from build123d import *

# Parameters (mm, degrees)
SKETCH_1_W                = 23.5
SKETCH_1_H                = 12
EXTRUDE_1_DEPTH           = 510.5
HOLE_WIZARD_M6_1_D        = 5
HOLE_WIZARD_M6_1_DEPTH    = 19
HOLE_WIZARD_M6_1_TIP      = 1.502151548
HOLE_WIZARD_M6_2_D        = 5
HOLE_WIZARD_M6_2_DEPTH    = 15
HOLE_WIZARD_M6_2_TIP      = 1.502151548
HOLE_WIZARD_9_0_9_1_D     = 9
HOLE_WIZARD_M6_3_D        = 5
HOLE_WIZARD_M6_3_DEPTH    = 15
HOLE_WIZARD_M6_3_TIP      = 1.502151548
HOLE_WIZARD_9_0_9_2_D     = 9
HOLE_WIZARD_7_0_7_1_D     = 7
HOLE_WIZARD_7_0_7_1_DEPTH = 15
HOLE_WIZARD_7_0_7_1_TIP   = 2.103012167
HOLE_WIZARD_M6_4_D        = 5
HOLE_WIZARD_M6_4_DEPTH    = 17
HOLE_WIZARD_M6_4_TIP      = 1.502151548


with BuildPart() as part:
    # 草图1 → 凸台-拉伸1 (new, symmetric)
    with BuildSketch(Plane(origin=(0, 0, 0), x_dir=(0, 0, -1), z_dir=(1, 0, 0))):
        Polygon((-15, 15), (-11.5, 15), (-11.5, 13.5), (-11, 13.5), (-11, 12), (-9.5, 12), (-9.5, 15), (-8, 15), (-8, 12.5), (-5, 12.5), (-5, 15), (5, 15), (5, 12.5), (8, 12.5), (8, 15), (9.5, 15), (9.5, 12), (11, 12), (11, 13.5), (11.5, 13.5), (11.5, 15), (15, 15), (15, 8), (12.5, 8), (12.5, 5), (15, 5), (15, -5), (12.5, -5), (12.5, -8), (15, -8), (15, -15), (11.5, -15), (11.5, -13.5), (11, -13.5), (11, -12), (9.5, -12), (9.5, -15), (8, -15), (8, -12.5), (5, -12.5), (5, -15), (-5, -15), (-5, -12.5), (-8, -12.5), (-8, -15), (-9.5, -15), (-9.5, -12), (-11, -12), (-11, -13.5), (-11.5, -13.5), (-11.5, -15), (-15, -15), align=None)
        with BuildLine():
            Line((12, -10.5), (12, -8.5))
            ThreePointArc((12, -8.5), (11.853553391, -8.146446609), (11.5, -8))
            Line((11.5, -8), (-11.5, -8))
            ThreePointArc((-11.5, -8), (-11.853553391, -8.146446609), (-12, -8.5))
            Line((-12, -8.5), (-12, -10.5))
            ThreePointArc((-12, -10.5), (-11.853553391, -10.853553391), (-11.5, -11))
            Line((-11.5, -11), (11.5, -11))
            ThreePointArc((11.5, -11), (11.853553391, -10.853553391), (12, -10.5))
        make_face(mode=Mode.SUBTRACT)
        with BuildLine():
            Line((-11.5, 11), (11.5, 11))
            ThreePointArc((11.5, 11), (11.853553391, 10.853553391), (12, 10.5))
            Line((12, 10.5), (12, 8.5))
            ThreePointArc((12, 8.5), (11.853553391, 8.146446609), (11.5, 8))
            Line((11.5, 8), (-11.5, 8))
            ThreePointArc((-11.5, 8), (-11.853553391, 8.146446609), (-12, 8.5))
            Line((-12, 8.5), (-12, 10.5))
            ThreePointArc((-12, 10.5), (-11.853553391, 10.853553391), (-11.5, 11))
        make_face(mode=Mode.SUBTRACT)
        Rectangle(SKETCH_1_W, SKETCH_1_H, mode=Mode.SUBTRACT)
    extrude(amount=EXTRUDE_1_DEPTH, both=True)

    # M6 螺纹孔1
    with Locations(Plane(origin=(0, 0, -15), x_dir=(-1, 0, 0), z_dir=(0, 0, -1))):
        with Locations((460.5, 0), (445.5, 0), (-445.5, 0), (-460.5, 0)):
            Hole(HOLE_WIZARD_M6_1_D / 2, depth=HOLE_WIZARD_M6_1_DEPTH)
            with Locations((0, 0, -(HOLE_WIZARD_M6_1_DEPTH + HOLE_WIZARD_M6_1_TIP / 2))):  # 118° drill point
                Cone(0, HOLE_WIZARD_M6_1_D / 2, HOLE_WIZARD_M6_1_TIP, mode=Mode.SUBTRACT)

    # M6 螺纹孔2
    with Locations(Plane(origin=(0, -15, 0), x_dir=(-1, 0, 0), z_dir=(0, -1, 0))):
        with Locations((-460.5, 0), (-445.5, 0), (215.5, 0), (230.5, 0), (445.5, 0), (460.5, 0)):
            Hole(HOLE_WIZARD_M6_2_D / 2, depth=HOLE_WIZARD_M6_2_DEPTH)
            with Locations((0, 0, -(HOLE_WIZARD_M6_2_DEPTH + HOLE_WIZARD_M6_2_TIP / 2))):  # 118° drill point
                Cone(0, HOLE_WIZARD_M6_2_D / 2, HOLE_WIZARD_M6_2_TIP, mode=Mode.SUBTRACT)

    # Ø9.0 (9) 直径孔1 (through all)
    with Locations(Plane.XY.offset(15)):
        with Locations((-422.5, 0), (422.5, 0)):
            Hole(HOLE_WIZARD_9_0_9_1_D / 2)

    # M6 螺纹孔3
    with Locations(Plane(origin=(0, 15, 0), x_dir=(1, 0, 0), z_dir=(0, 1, 0))):
        with Locations((-355.5, 0), (400.5, 0)):
            Hole(HOLE_WIZARD_M6_3_D / 2, depth=HOLE_WIZARD_M6_3_DEPTH)
            with Locations((0, 0, -(HOLE_WIZARD_M6_3_DEPTH + HOLE_WIZARD_M6_3_TIP / 2))):  # 118° drill point
                Cone(0, HOLE_WIZARD_M6_3_D / 2, HOLE_WIZARD_M6_3_TIP, mode=Mode.SUBTRACT)

    # Ø9.0 (9) 直径孔2 (through all)
    with Locations(Plane(origin=(0, -15, 0), x_dir=(-1, 0, 0), z_dir=(0, -1, 0))):
        with Locations((-183, 0), (390.5, 0)):
            Hole(HOLE_WIZARD_9_0_9_2_D / 2)

    # Ø7.0 (7) 直径孔1
    with Locations(Plane(origin=(0, -15, 0), x_dir=(-1, 0, 0), z_dir=(0, -1, 0))):
        with Locations((-400.5, 0), (355.5, 0)):
            Hole(HOLE_WIZARD_7_0_7_1_D / 2, depth=HOLE_WIZARD_7_0_7_1_DEPTH)
            with Locations((0, 0, -(HOLE_WIZARD_7_0_7_1_DEPTH + HOLE_WIZARD_7_0_7_1_TIP / 2))):  # 118° drill point
                Cone(0, HOLE_WIZARD_7_0_7_1_D / 2, HOLE_WIZARD_7_0_7_1_TIP, mode=Mode.SUBTRACT)

    # M6 螺纹孔4
    with Locations(Plane(origin=(0, 0, -15), x_dir=(-1, 0, 0), z_dir=(0, 0, -1))):
        with Locations((-368.5, 0), (-298.499999898, 0)):
            Hole(HOLE_WIZARD_M6_4_D / 2, depth=HOLE_WIZARD_M6_4_DEPTH)
            with Locations((0, 0, -(HOLE_WIZARD_M6_4_DEPTH + HOLE_WIZARD_M6_4_TIP / 2))):  # 118° drill point
                Cone(0, HOLE_WIZARD_M6_4_D / 2, HOLE_WIZARD_M6_4_TIP, mode=Mode.SUBTRACT)


solid = part.part
The model under review builds one solid part; all positions refer to its coordinate system, in mm. A direction names the side the tool comes from. Round coordinates to 2 decimals unless told otherwise and drop trailing zeros. Answer as CSV lines item,"result".
1. Insertion check: pin 1 Ø8 at (x, y) = (298.5, 0) entering from -Z; pin 2 Ø3 at (x, z) = (-355.5, 0) entering from +Y. Each pin has a flat end and moves straight along its axis. Give the tip position at first contact, or say it passes through.
Outcome:
pin 1,"stops at z = -15"
pin 2,"passes through"
2. We need section A-A (x = -43.5). Count the separate pieces of the cut face and the enclosed holes in it, plus the area to 3 significant figures.
Outcome:
separate pieces,"1"
enclosed holes,"3"
area,"408 mm2"
3. To check wall thickness, follow L1, parallel to Y at x = 226.5, z = -4.5; L2, parallel to Y at x = -434.5, z = -13; L3, parallel to Y at x = -414.5, z = 7.25. State the ranges of each line that lie inside material, in increasing order. Write a range as [from, to].
Outcome:
L1,"y = [-15, -11], [-8, -6], [6, 8], [11, 15]"
L2,"y = [-15, -8], [-5, 5], [8, 15]"
L3,"y = [-12.5, -11], [-8, -6], [6, 8], [11, 12.5]"
4. Draft analysis for pull direction Z (two halves, no side actions). For faces 3 (the face through (510.5, 7, 0)), 4 (the face through (7, 8, 0)), 5 (the face through (7, 0, 15)), state which applies: pulls with the +Z half, pulls with the -Z half, needs draft (parallel to the pull), parting line crosses it, or undercut.
Outcome:
face 3,"needs draft"
face 4,"undercut"
face 5,"pulls with the +Z half"
5. For faces 1 (the face through (-510.5, 7, 0)), 2 (the face through (7, -11, 0)), list the 3-axis set-ups (+Z, -Z, +X, -X, +Y, -Y) from which the entire face can be reached by the end or side of a thin tool; tool diameter is ignored.
Outcome:
face 1,"+Z, -Z, -X, +Y, -Y"
face 2,"+X, -X"
